Design review of the part built by this model. Coordinates are the model's own, in mm. A direction names the side the tool comes from. Coordinates: 2 decimals unless noted, no trailing zeros. Write each loop counter-clockwise with the first axis right and the second up, starting at its lowest first coordinate (ties: lowest second). Pieces come first, ordered by that corner, then holes. Notation, with made-up numbers: (5, -2.5) -> (26, -2.5) arc R16 ccw to (26, 7.5) -> close; hole circle Ø1 at (77.5, 72.5). An arc over 180 degrees is marked (long way). One line per question, with ' | ' between items. Start each with the question number.
Q1. Add section B-B on x = -35.5. State the section outline as (y, z) points.
Q2. Add section D-D on z = -16.5. State the section outline as (x, y) points.
Q3. For faces 5 (the flat face through (-20.3, 2.6, -4.3)), 6 (the cylindrical face through (2.74, 2.09, -17.29)), 7 (the flat face through (24, 1.3, 32)), list the 3-axis set-ups (+Z, -Z, +X, -X, +Y, -Y) from which the entire face can be reached by the end or side of a thin tool; tool diameter is ignored.
Q4. For P1, Ø7.5, axis at x = -38, z = 19.5, coming from the +Y side; P2, Ø1.6, axis at x = -48.5, z = -21.5, coming from the +Y side, all flat-tipped, find the tip position at first contact; note any pin that passes through.
Q5. Add section A-A on z = 21. State the section outline as (x, y) points.
Q6. Draft analysis for pull direction Z (two halves, no side actions). For faces 1 (the cylindrical face through (-41.05, 2.09, -19.28)), 2 (the flat face through (-48, 1.3, -21)), 3 (the flat face through (10, 1.6, 18)), 4 (the flat face through (-13, 1, 33.73)), state which applies: pulls with the +Z half, pulls with the -Z half, needs draft (parallel to the pull), parting line crosses it, or undercut.
Q7. Add section C-C on x = -17. State the section outline as (y, z) points.
Q8. Wall thickness on probe 1 along Z at (x, y) = (21, 2.3); probe 2 along Z at (x, y) = (15.5, 2.35); probe 3 along X at (y, z) = (2.5, 21.5) (3 decimals): over which ranges is each line inside the solid? List them lowest first.
from build123d import *

# Parameters (mm, degrees)
SKETCH1_W           = 75.233320997
SKETCH1_H           = 56.2
BOSS_EXTRUDE1_DEPTH = 1.6
SKETCH2_R           = 13.5
SKETCH2_R_2         = 12.5
BOSS_EXTRUDE2_DEPTH = 1
SKETCH3_W           = 3.2
SKETCH3_H           = 3.2
CUT_EXTRUDE1_DEPTH  = 0.3


with BuildPart() as part:
    # Sketch1 → Boss-Extrude1 (new body)
    with BuildSketch(Plane(origin=(0, 0, 0), x_dir=(1, 0, 0), z_dir=(0, 1, 0))):
        with Locations((-12.172352394, -5.629712982)):
            Rectangle(SKETCH1_W, SKETCH1_H)
    extrude(amount=BOSS_EXTRUDE1_DEPTH)

    # Sketch2 → Boss-Extrude2 (add)
    # profile 1 of 5: a face of its own
    with BuildSketch(Plane(origin=(0, 1.6, 0), x_dir=(1, 0, 0), z_dir=(0, 1, 0))):
        with Locations((10.344308105, 7.370287018)):
            Circle(SKETCH2_R)
        with Locations(Location((10.344308105, 7.370287018, 0), (0, 0, 270))):
            Circle(SKETCH2_R_2, mode=Mode.SUBTRACT)
    # profile 2 of 5: a face of its own
    with BuildSketch(Plane(origin=(0, 1.6, 0), x_dir=(1, 0, 0), z_dir=(0, 1, 0))):
        with Locations((10.344308105, -18.629712982)):
            Circle(SKETCH2_R)
        with Locations(Location((10.344308105, -18.629712982, 0), (0, 0, 270))):
            Circle(SKETCH2_R_2, mode=Mode.SUBTRACT)
    # profile 3 of 5: a face of its own
    with BuildSketch(Plane(origin=(0, 1.6, 0), x_dir=(1, 0, 0), z_dir=(0, 1, 0))):
        with Locations((-12.172352394, -5.629712982)):
            Circle(SKETCH2_R)
        with Locations(Location((-12.172352394, -5.629712982, 0), (0, 0, 270))):
            Circle(SKETCH2_R_2, mode=Mode.SUBTRACT)
    # profile 4 of 5: a face of its own
    with BuildSketch(Plane(origin=(0, 1.6, 0), x_dir=(1, 0, 0), z_dir=(0, 1, 0))):
        with Locations((-34.689012892, 7.370287018)):
            Circle(SKETCH2_R)
        with Locations(Location((-34.689012892, 7.370287018, 0), (0, 0, 270))):
            Circle(SKETCH2_R_2, mode=Mode.SUBTRACT)
    # profile 5 of 5: a face of its own
    with BuildSketch(Plane(origin=(0, 1.6, 0), x_dir=(1, 0, 0), z_dir=(0, 1, 0))):
        with Locations((-34.689012892, -18.629712982)):
            Circle(SKETCH2_R)
        with Locations(Location((-34.689012892, -18.629712982, 0), (0, 0, 270))):
            Circle(SKETCH2_R_2, mode=Mode.SUBTRACT)
    extrude(amount=BOSS_EXTRUDE2_DEPTH)

    # Sketch3 → Cut-Extrude1 (cut)
    with BuildSketch(Plane(origin=(0, 1.6, 0), x_dir=(1, 0, 0), z_dir=(0, 1, 0))):
        with Locations((-48.189012892, -32.129712982)):
            Rectangle(SKETCH3_W, SKETCH3_H)
        with Locations((23.844308105, -32.129712982)):
            Rectangle(SKETCH3_W, SKETCH3_H)
        with Locations((23.844308105, 20.870287018)):
            Rectangle(SKETCH3_W, SKETCH3_H)
        with Locations((-48.189012892, 20.870287018)):
            Rectangle(SKETCH3_W, SKETCH3_H)
    extrude(amount=-CUT_EXTRUDE1_DEPTH, mode=Mode.SUBTRACT)


solid = part.part
Output values:
1) outline: (0, -22.47) -> (1.6, -22.47) -> (1.6, -20.85) -> (2.6, -20.85) -> (2.6, -19.84) -> (1.6, -19.84) -> (1.6, 5.1) -> (2.6, 5.1) -> (2.6, 6.16) -> (1.6, 6.16) -> (1.6, 31.1) -> (2.6, 31.1) -> (2.6, 32.11) -> (1.6, 32.11) -> (1.6, 33.73) -> (0, 33.73) -> close
2) outline: (-49.79, 0) -> (25.44, 0) -> (25.44, 1.6) -> (20.29, 1.6) -> (20.29, 2.6) -> (18.88, 2.6) -> (18.88, 1.6) -> (1.81, 1.6) -> (1.81, 2.6) -> (0.4, 2.6) -> (0.4, 1.6) -> (-24.74, 1.6) -> (-24.74, 2.6) -> (-26.15, 2.6) -> (-26.15, 1.6) -> (-43.23, 1.6) -> (-43.23, 2.6) -> (-44.63, 2.6) -> (-44.63, 1.6) -> (-49.79, 1.6) -> close
3) face 5: +Z, -Z, +X, -X, +Y | face 6: +Y | face 7: +Z, +X, +Y
4) P1: stops at y = 1.6 | P2: stops at y = 1.3
5) outline: (-49.79, 0) -> (25.44, 0) -> (25.44, 1.6) -> (23.63, 1.6) -> (23.63, 2.6) -> (22.62, 2.6) -> (22.62, 1.6) -> (-1.93, 1.6) -> (-1.93, 2.6) -> (-2.95, 2.6) -> (-2.95, 1.6) -> (-21.4, 1.6) -> (-21.4, 2.6) -> (-22.42, 2.6) -> (-22.42, 1.6) -> (-46.96, 1.6) -> (-46.96, 2.6) -> (-47.98, 2.6) -> (-47.98, 1.6) -> (-49.79, 1.6) -> close
6) face 1: undercut | face 2: needs draft | face 3: undercut | face 4: pulls with the +Z half
7) outline: (0, -22.47) -> (1.6, -22.47) -> (1.6, -6.98) -> (2.6, -6.98) -> (2.6, -5.9) -> (1.6, -5.9) -> (1.6, 17.16) -> (2.6, 17.16) -> (2.6, 18.24) -> (1.6, 18.24) -> (1.6, 33.73) -> (0, 33.73) -> close
8) probe 1: z = -15.66 to -13.91, -0.84 to 0.92, 10.34 to 12.09, 25.16 to 26.92 | probe 2: z = -19.85 to -18.76, 4.02 to 5.11, 6.15 to 7.24, 30.02 to 31.11 | probe 3: x = -47.88 to -46.855, -22.523 to -21.498, -2.847 to -1.822, 22.51 to 23.536
